from build123d import *

# Parameters (mm, degrees)
F2_R          = 5.05
F3_DEPTH      = 3
F0_R          = 4.5
F4_DEPTH      = 3
F5_DEPTH      = 7
F8_DEPTH      = 3
F9_DEPTH      = 1
F9_DEPTH_BACK = 1


with BuildPart() as f3:
    # F2 (on offset) → F3 (new body)
    with BuildSketch(Plane.XY.offset(3.3)):
        with BuildLine():
            ThreePointArc((-3, -31.5561521365), (-3.1464466094, -31.2025987459), (-3.5, -31.0561521365))
            Line((-3.5, -31.0561521365), (-3.5, -31.5561521365))
            Line((-3.5, -31.5561521365), (-3, -31.5561521365))
        make_face()
        with BuildLine():
            Line((3.5, -6.6332495807), (3.5, -5.5217424324))
            Line((3.5, -5.5217424324), (-3.5, -5.5217424324))
            Line((-3.5, -5.5217424324), (-3.5, -6.6332495807))
            Line((-3.5, -6.6332495807), (-3.5, -31.0561521365))
            ThreePointArc((-3.5, -31.0561521365), (-3.1464466094, -31.2025987459), (-3, -31.5561521365))
            Line((-3, -31.5561521365), (3.5, -31.5561521365))
            Line((3.5, -31.5561521365), (3.5, -6.6332495807))
        make_face()
        with BuildLine():
            Line((-3.5, -5.5217424324), (3.5, -5.5217424324))
            Line((3.5, -5.5217424324), (3.5, -6.6332495807))
            ThreePointArc((3.5, -6.6332495807), (0, 7.5), (-3.5, -6.6332495807))
            Line((-3.5, -6.6332495807), (-3.5, -5.5217424324))
        make_face()
        Circle(F2_R, mode=Mode.SUBTRACT)
    extrude(amount=F3_DEPTH)



with BuildPart() as f4:
    # F0 (on Top) → F4 (new body)
    with BuildSketch(Plane.XY):
        Polygon((3.5, -31.5561521365), (3.5, -6.6332495807), (3.5, -5.5217424324), (-3.5, -5.5217424324), (-3.5, -6.6332495807), (-3.5, -31.5561521365), align=None)
        with BuildLine():
            Line((3.5, -5.5217424324), (3.5, -6.6332495807))
            ThreePointArc((3.5, -6.6332495807), (0, 7.5), (-3.5, -6.6332495807))
            Line((-3.5, -6.6332495807), (-3.5, -5.5217424324))
            Line((-3.5, -5.5217424324), (3.5, -5.5217424324))
        make_face()
        Circle(F0_R, mode=Mode.SUBTRACT)
        Circle(F0_R)
    extrude(amount=F4_DEPTH)

    # F0 (on Top) → F5 (join)
    with BuildSketch(Plane.XY):
        Circle(F0_R)
    extrude(amount=F5_DEPTH)

    # F7 (on offset) → F8 (join)
    with BuildSketch(Plane.XY.offset(7)):
        with BuildLine():
            Line((-3.5, -6.6332495807), (3.5, -6.6332495807))
            ThreePointArc((3.5, -6.6332495807), (0, 7.5), (-3.5, -6.6332495807))
        make_face()
    extrude(amount=F8_DEPTH)


with BuildPart() as f3_1:
    add(f3.part)

    add(f4.part)  # F9 merges F4
    # F2 (on offset) → F9 (join, two sides)
    with BuildSketch(Plane.XY.offset(3.3)) as f9_sk:
        with BuildLine():
            Line((-3.5, -31.5561521365), (-3.5, -31.0561521365))
            ThreePointArc((-3.5, -31.0561521365), (-3.8535533906, -31.9097055271), (-3, -31.5561521365))
            Line((-3, -31.5561521365), (-3.5, -31.5561521365))
        make_face()
    extrude(amount=F9_DEPTH)
    extrude(f9_sk.sketch, amount=-F9_DEPTH_BACK)


solid = f3_1.part
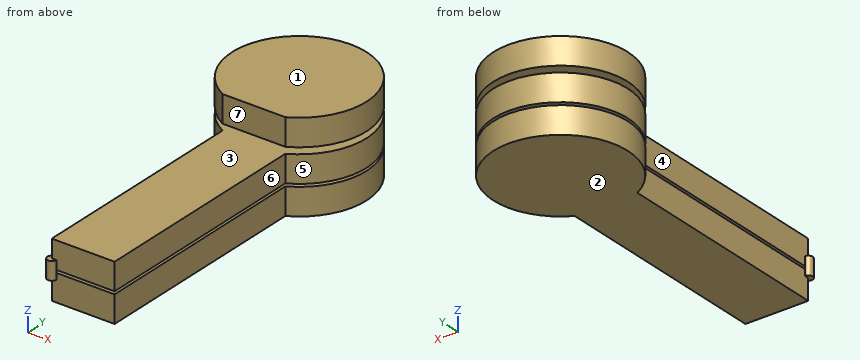
Can you work these out from the model? Positions are in its coordinate system, mm. Face numbers are marked on the shaded views. A direction names the side the tool comes from. Give positions to 0.01 mm unless a question says otherwise; leave off trailing zeros. Order: outer loops, then holes, each group sorted by start corner. A loop starts at its lowest first (then second) coordinate and runs counter-clockwise, first axis right, second up. Notation, with made-up numbers: M 9.5,-21.5 L 23.5,-21.5 A12 ccw 23.5,1.5 Z; hole C 71,21.5 d9. An arc over 180 degrees is marked long. Use one line per item in the form item = value. Start each with the question number.
Item 1: If I drill on line 1 along Y through (x, z) = (0, 4.05); line 2 along Z through (x, y) = (5.75, -0.5); line 3 along Z through (x, y) = (1.25, -20), over which ranges is the centre line in solid material (lowest first)?
Item 2: We'd pull the mould along Z, two halves only. Please class the marked faces 1, 2, 3 and 4: +Z half, -Z half, draft (parallel to the pull), parting line (faces both ways), or undercut.
Item 3: For the marked faces 5, 6 and 7, which set-ups out of +Z, -Z, +X, -X, +Y, -Y let a thin tool reach every point of the face, with its end or its side?
Item 4: Will these pins go through, and if not, where does the flat tip stop? pin 1 Ø2.5 at (y, z) = (-23, 2) entering from -X; pin 2 Ø2.5 at (y, z) = (-24.5, 5) entering from +X; pin 3 Ø2.5 at (x, z) = (0.5, 1) entering from -Y.
Item 5: If we section it at C-C (y = -27): Write out the boundary of the cut face in (x, z), then the cut area to 3 significant figures.
Item 6: If we section it at A-A (y = 0): Write out the boundary of the cut face in (x, z).
Item 7: If we section it at B-B (x = 0): Write out the boundary of the cut face in (y, z), then the cut area to 3 significant figures.
Item 8: If we section it at D-D (z = 1): Write out the boundary of the cut face in (x, y), then the cut area to 3 significant figures.
Outcome:
q1.line_1 = -31.56 to -5.05, -4.5 to 4.5, 5.05 to 7.5
q1.line_2 = 0 to 3, 3.3 to 6.3, 7 to 10
q1.line_3 = 0 to 3, 3.3 to 6.3
q2.face_1 = +Z half
q2.face_2 = -Z half
q2.face_3 = undercut
q2.face_4 = draft
q3.face_5 = +Z, -Z
q3.face_6 = +Z, -Z, +X, -Y
q3.face_7 = +Z, +X, -X, -Y
q4.pin_1 = -3.5
q4.pin_2 = 3.5
q4.pin_3 = -31.56
q5.outline = M -3.5,0 L 3.5,0 L 3.5,3 L -3.5,3 Z; M -3.5,3.3 L 3.5,3.3 L 3.5,6.3 L -3.5,6.3 Z
q5.area = 42.0 mm2
q6.outline = M -7.5,0 L 7.5,0 L 7.5,3 L 4.5,3 L 4.5,7 L 7.5,7 L 7.5,10 L -7.5,10 L -7.5,7 L -4.5,7 L -4.5,3 L -7.5,3 Z; M -7.5,3.3 L -5.05,3.3 L -5.05,6.3 L -7.5,6.3 Z; M 5.05,3.3 L 7.5,3.3 L 7.5,6.3 L 5.05,6.3 Z
q7.outline = M -31.56,0 L 7.5,0 L 7.5,3 L 4.5,3 L 4.5,7 L 7.5,7 L 7.5,10 L -6.63,10 L -6.63,7 L -4.5,7 L -4.5,3 L -31.56,3 Z; M -31.56,3.3 L -5.05,3.3 L -5.05,6.3 L -31.56,6.3 Z; M 5.05,3.3 L 7.5,3.3 L 7.5,6.3 L 5.05,6.3 Z
q7.area = 282 mm2
q8.outline = M -3.5,-31.56 L 3.5,-31.56 L 3.5,-6.63 A7.5 ccw long -3.5,-6.63 Z
q8.area = 347 mm2
